from build123d import *

# Parameters (mm, degrees)
F0_W     = 774.7
F0_H     = 76.2
F1_DEPTH = 5.9944
F2_R     = 6.35
F3_DEPTH = 11.9888
F4_R     = 6.35
F5_DEPTH = 11.9888
F6_W     = 177.8
F6_H     = 76.2
F7_DEPTH = 11.9888


with BuildPart() as f1:
    # F0 (on Top) → F1 (new body, symmetric)
    with BuildSketch(Plane.XY):
        Rectangle(F0_W, F0_H)
    extrude(amount=F1_DEPTH, both=True)

    # F2 (on face) → F3 (cut, through all)
    with BuildSketch(Plane(origin=(0, 0, -5.9944), x_dir=(1, 0, 0), z_dir=(0, 0, -1))):
        with Locations((-316.70625, 0)):
            Circle(F2_R)
        with Locations((323.85, 0)):
            Circle(F2_R)
    extrude(amount=-F3_DEPTH, mode=Mode.SUBTRACT)

    # F4 (on face) → F5 (cut, through all)
    with BuildSketch(Plane.XY.offset(5.9944)):
        with Locations((-349.25, 0)):
            Circle(F4_R)
        with Locations((-234.95, 0)):
            Circle(F4_R)
    extrude(amount=-F5_DEPTH, mode=Mode.SUBTRACT)

    # F6 (on face) → F7 (cut, through all)
    with BuildSketch(Plane.XY.offset(5.9944)):
        with Locations((-298.45, 0)):
            Rectangle(F6_W, F6_H)
    extrude(amount=-F7_DEPTH, mode=Mode.SUBTRACT)


solid = f1.part
Here's how the part is built. I have some questions about the finished solid (model axes, mm). Round coordinates to 2 decimals unless told otherwise and drop trailing zeros. Write each loop counter-clockwise with the first axis right and the second up, starting at its lowest first coordinate (ties: lowest second). Pieces come first, ordered by that corner, then holes.
1. If we mould it in two halves opening along X, with no side actions, what happens to faces 1 (the flat face through (-209.55, -1, 0)), 2 (the flat face through (387.35, -1, 0)), 3 (the flat face through (85, 1, -5.994)), 4 (the cylindrical face through (329.716, 2.432, -0.084))? For each: released by +X, released by -X, zero draft, split by the parting line, or undercut.
2. Suppose I cut it at A-A (x = 323.85). List the corners of the cut face in (y, z) for me, and give its area (3 significant figures).
3. I need wall thicknesses on L1, parallel to X at y = 0, z = 0.5; L2, parallel to Y at x = 323.85, z = 1; L3, parallel to X at y = -3.5, z = 0.5. Which ranges of each line are inside material? Lowest first, please.
4. Suppose I cut it at B-B (y = 0). List the corners of the cut face in (x, z) for me, and give its area (3 significant figures).
Answer sheet:
1. face 1: released by -X
1. face 2: released by +X
1. face 3: zero draft
1. face 4: undercut
2. outline: (-38.1, -5.99) - (-6.35, -5.99) - (-6.35, 5.99) - (-38.1, 5.99) - close; (6.35, -5.99) - (38.1, -5.99) - (38.1, 5.99) - (6.35, 5.99) - close
2. area: 761 mm2
3. L1: x = -209.55 to 317.5, 330.2 to 387.35
3. L2: y = -38.1 to -6.35, 6.35 to 38.1
3. L3: x = -209.55 to 318.55, 329.15 to 387.35
4. outline: (-209.55, -5.99) - (317.5, -5.99) - (317.5, 5.99) - (-209.55, 5.99) - close; (330.2, -5.99) - (387.35, -5.99) - (387.35, 5.99) - (330.2, 5.99) - close
4. area: 7,000 mm2
